Input: dimensioned drawing with shaded views. Units: mm. Origin: part minimum x, y, z. A direction names the side the tool comes from. Round coordinates to 2 decimals unless told otherwise and drop trailing zeros. Order: outer loops, then holes, each group sorted by start corner. A loop starts at its lowest first (then second) coordinate and runs counter-clockwise, first axis right, second up. Notation, with made-up numbers: M 37,74.25 L 65,74.25 A11 cw 65,78.25 Z; hole C 18.25,86 d3. An arc over 180 degrees is marked long. Put each result on its own line as item: value. Start each with the question number.
1) Section C-C, the plane y = 35. Return loops of the section in (x, z).
2) Section A-A, the plane x = 23. Return loops of the section in (y, z).
3) Access query for the marked faces 5, 6, 7 and 8. Directions: +Z, -Z, +X, -X, +Y, -Y. A direction counts if a zero-diameter tool reaches every point of the face in a straight line with its end or side. Return the directions, or none.
4) Draft query along Z for the marked faces 1, 2, 3 and 4. Return one class per face: pulls with the +Z half, pulls with the -Z half, needs draft (parallel to the pull), parting line crosses it, or undercut.
5) Material intervals for probe 1 along Y at (x, z) = (23, 2); probe 2 along X at (y, z) = (20, 2.25); probe 3 along Z at (x, y) = (32, 8), sorted ascending. Write a range as [from, to].
6) First-contact query: P1, Ø1, axis at y = 12.5, z = 11.5, coming from the +X side; P2, Ø5, axis at x = 23, y = 20, coming from the +Z side; P3, Ø12, axis at x = 63, z = 25, coming from the -Y side; P4, Ø4, axis at x = 56, z = 23, coming from the +Y side. Flat tips, straight axial feed; report the tip coordinate or a pass-through.
7) Section D-D, the plane y = 14.5. Return loops of the section in (x, z).
8) Section B-B, the plane z = 12. Return loops of the section in (x, y), then the cut area to 3 significant figures.
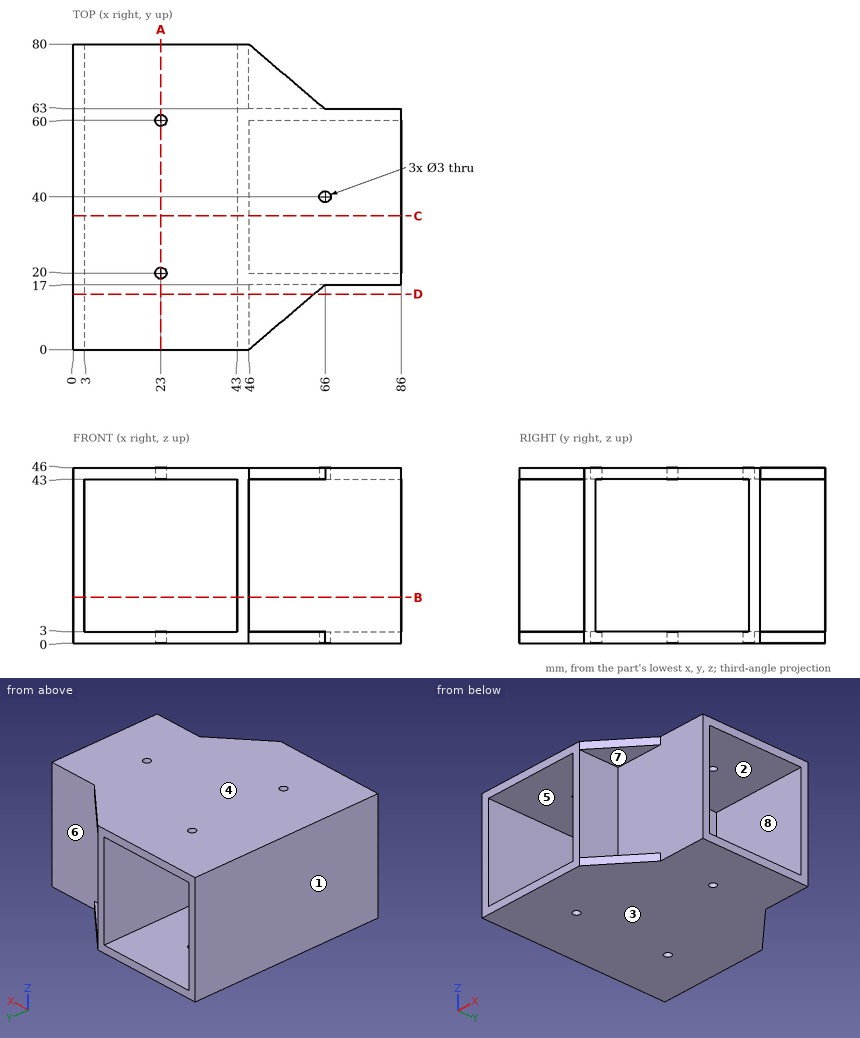
Result sheet:
1. outline: M 0,0 L 86,0 L 86,3 L 46,3 L 46,43 L 86,43 L 86,46 L 0,46 Z; hole M 3,3 L 43,3 L 43,43 L 3,43 Z
2. outline: M 0,0 L 18.5,0 L 18.5,3 L 0,3 Z; M 0,43 L 18.5,43 L 18.5,46 L 0,46 Z; M 21.5,0 L 58.5,0 L 58.5,3 L 21.5,3 Z; M 21.5,43 L 58.5,43 L 58.5,46 L 21.5,46 Z; M 61.5,0 L 80,0 L 80,3 L 61.5,3 Z; M 61.5,43 L 80,43 L 80,46 L 61.5,46 Z
3. face 5: +Y, -Y
3. face 6: +X, +Y
3. face 7: +X, -Y
3. face 8: +X
4. face 1: needs draft
4. face 2: undercut
4. face 3: pulls with the -Z half
4. face 4: pulls with the +Z half
5. probe 1: y = [0, 18.5], [21.5, 58.5], [61.5, 80]
5. probe 2: x = [0, 21.5], [24.5, 86]
5. probe 3: z = [0, 3], [43, 46]
6. P1: stops at x = 46
6. P2: stops at z = 46
6. P3: stops at y = 17
6. P4: stops at y = 63
7. outline: M 0,0 L 63.06,0 L 63.06,3 L 46,3 L 46,43 L 63.06,43 L 63.06,46 L 0,46 Z; hole M 3,3 L 43,3 L 43,43 L 3,43 Z
8. outline: M 0,0 L 3,0 L 3,80 L 0,80 Z; M 43,0 L 46,0 L 46,17 L 86,17 L 86,20 L 46,20 L 46,60 L 86,60 L 86,63 L 46,63 L 46,80 L 43,80 Z
8. area: 720 mm2
